Check sheet for the modelled part. Datum: model origin and axes. Units: mm. A direction names the side the tool comes from. Round coordinates to 2 decimals unless told otherwise and drop trailing zeros. Write each loop counter-clockwise with the first axis right and the second up, starting at its lowest first coordinate (ties: lowest second). Pieces come first, ordered by that corner, then holes. Notation, with made-up numbers: M 75,26 L 84,26 A18 ccw 84,54 Z; hole C 28,17.25 d9. An arc over 180 degrees is marked long. Put each result on its own line as item: value.
```python
from build123d import *

# Parameters (mm, degrees)
SKETCH1_W            = 4.8
SKETCH1_H            = 4.8
BOSS_EXTRUDE1_DEPTH  = 20
SKETCH2_W            = 5.2
SKETCH2_H            = 5.2
BOSS_EXTRUDE2_DEPTH  = 50
SKETCH3_W            = 17
SKETCH3_H            = 27
BOSS_EXTRUDE3_DEPTH  = 10
SKETCH4_W            = 13
SKETCH4_H            = 23
CUT_EXTRUDE1_DEPTH   = 8.5
SKETCH5_W            = 11
SKETCH5_H            = 8.5
CUT_EXTRUDE2_DEPTH   = 8.5
SKETCH6_W            = 5
SKETCH6_H            = 5
BOSS_EXTRUDE4_DEPTH  = 81.5
SKETCH7_W            = 5
SKETCH7_H            = 5
BOSS_EXTRUDE5_DEPTH  = 43.1
SKETCH9_R            = 0.9
CUT_EXTRUDE4_DEPTH   = 125.748466924
BOSS_EXTRUDE6_DEPTH  = 5.2
SKETCH13_W           = 17
SKETCH13_H           = 27
BOSS_EXTRUDE7_DEPTH  = 1.5
SKETCH14_W           = 17
SKETCH14_H           = 27
SKETCH14_W_2         = 13
SKETCH14_H_2         = 23
BOSS_EXTRUDE8_DEPTH  = 8.5
SKETCH15_W           = 11
SKETCH15_H           = 8.5
CUT_EXTRUDE6_DEPTH   = 8.5
BOSS_EXTRUDE9_REACH  = 100.782
SKETCH16_W           = 5
SKETCH16_H           = 5
BOSS_EXTRUDE10_DEPTH = 5.2


with BuildPart() as part:
    # Sketch1 → Boss-Extrude1 (new body)
    with BuildSketch(Plane.XY):
        with Locations((2.4, -2.4)):
            Rectangle(SKETCH1_W, SKETCH1_H)
    extrude(amount=BOSS_EXTRUDE1_DEPTH)

    # Sketch2 → Boss-Extrude2 (add)
    with BuildSketch(Plane(origin=(0, 0, 0), x_dir=(-1, 0, 0), z_dir=(0, 0, -1))):
        with Locations((-2.4, -2.4)):
            Rectangle(SKETCH2_W, SKETCH2_H)
    extrude(amount=BOSS_EXTRUDE2_DEPTH)

    # Sketch3 → Boss-Extrude3 (add)
    with BuildSketch(Plane(origin=(0, 0, -50), x_dir=(-1, 0, 0), z_dir=(0, 0, -1))):
        with Locations((-2.4, -2.4)):
            Rectangle(SKETCH3_W, SKETCH3_H)
    extrude(amount=BOSS_EXTRUDE3_DEPTH)

    # Sketch4 → Cut-Extrude1 (cut)
    with BuildSketch(Plane(origin=(0, 0, -60), x_dir=(-1, 0, 0), z_dir=(0, 0, -1))):
        with Locations((-2.4, -2.4)):
            Rectangle(SKETCH4_W, SKETCH4_H)
    extrude(amount=-CUT_EXTRUDE1_DEPTH, mode=Mode.SUBTRACT)

    # Sketch5 → Cut-Extrude2 (cut)
    with BuildSketch(Plane.XZ.offset(15.9)):
        with Locations((2.4, -54.25)):
            Rectangle(SKETCH5_W, SKETCH5_H)
    extrude(amount=-CUT_EXTRUDE2_DEPTH, mode=Mode.SUBTRACT)

    # Sketch6 → Boss-Extrude4 (add)
    with BuildSketch(Plane(origin=(0, 0.2, 0), x_dir=(1, 0, 0), z_dir=(0, 1, 0))):
        with Locations((2.4, 37.5)):
            Rectangle(SKETCH6_W, SKETCH6_H)
    extrude(amount=-BOSS_EXTRUDE4_DEPTH)

    # Sketch7 → Boss-Extrude5 (add)
    with BuildSketch(Plane(origin=(0, 0, -40), x_dir=(-1, 0, 0), z_dir=(0, 0, -1))):
        with Locations((-2.4, -78.8)):
            Rectangle(SKETCH7_W, SKETCH7_H)
    extrude(amount=BOSS_EXTRUDE5_DEPTH)

    # Sketch9 → Cut-Extrude4 (cut, through all)
    with BuildSketch(Plane.XZ.offset(81.3)):
        with Locations((2.4, -80.1)):
            Circle(SKETCH9_R)
    extrude(amount=-CUT_EXTRUDE4_DEPTH, mode=Mode.SUBTRACT)

    # Sketch12 → Boss-Extrude6 (add)
    with BuildSketch(Plane(origin=(5, 0, 0), x_dir=(0, 0, -1), z_dir=(1, 0, 0))):
        Polygon((13.455782968, -5), (35, -40.359932103), (35, -45.359932103), (8.455782968, -5), align=None)
    extrude(amount=-BOSS_EXTRUDE6_DEPTH)


with BuildPart() as body_2:
    # Sketch13 → Boss-Extrude7 (new body)
    with BuildSketch(Plane(origin=(0, -54.71, 0), x_dir=(-1, 0, 0), z_dir=(0, -1, 0))):
        with Locations((-2.6, 15.4)):
            Rectangle(SKETCH13_W, SKETCH13_H)
    extrude(amount=BOSS_EXTRUDE7_DEPTH)

    # Sketch14 → Boss-Extrude8 (add)
    with BuildSketch(Plane.XZ.offset(56.21)):
        with Locations((2.6, -15.4)):
            Rectangle(SKETCH14_W, SKETCH14_H)
        with Locations((2.6, -15.4)):
            Rectangle(SKETCH14_W_2, SKETCH14_H_2, mode=Mode.SUBTRACT)
    extrude(amount=BOSS_EXTRUDE8_DEPTH)

    # Sketch15 → Cut-Extrude6 (cut)
    with BuildSketch(Plane.XY.offset(-1.9)):
        with Locations((2.6, -58.96)):
            Rectangle(SKETCH15_W, SKETCH15_H)
    extrude(amount=-CUT_EXTRUDE6_DEPTH, mode=Mode.SUBTRACT)

    # Sketch16 → Boss-Extrude9 (add, up to next)
    with BuildSketch(Plane.XY.offset(-35), mode=Mode.PRIVATE) as boss_extrude9_sk1:
        with Locations((2.4, -59.859932103)):
            Rectangle(SKETCH16_W, SKETCH16_H)
    boss_extrude9_tool1 = extrude(boss_extrude9_sk1.sketch, amount=BOSS_EXTRUDE9_REACH, mode=Mode.PRIVATE) - body_2.part

    add(part.part)  # Boss-Extrude9 merges part
    add(boss_extrude9_tool1.solids().sort_by_distance((2.4, -59.859932, -35))[0])

    # Sketch18 → Boss-Extrude10 (add)
    with BuildSketch(Plane(origin=(0, 0, 0), x_dir=(0, 0, -1), z_dir=(1, 0, 0))):
        Polygon((25.666047821, -54.71), (5.38231876, -5), (0.38231876, -5), (20.666047821, -54.71), align=None)
    extrude(amount=BOSS_EXTRUDE10_DEPTH)


solid = body_2.part
```
1. Cross-section at D-D (z = 3.5). Enter the section's corners in (x, y), then the cut area to 3 significant figures.
Computed values:
outline: M 0,-4.8 L 4.8,-4.8 L 4.8,0 L 0,0 Z
area: 23.0 mm2
2. Cross-section at B-B (y = -18). Enter the section's corners in (x, z), then the cut area to 3 significant figures.
Computed values:
outline: M -0.2,-21.38 L 5,-21.38 L 5,-17.01 L -0.2,-17.01 Z; M -0.1,-40 L 4.9,-40 L 4.9,-35 L -0.1,-35 Z; M 0,-10.69 L 5.2,-10.69 L 5.2,-5.69 L 0,-5.69 Z
area: 73.7 mm2
3. Depth check by flat-ended pin: pin 1 Ø2.5 at (x, z) = (3.5, 7) entering from -Y; pin 2 Ø1.5 at (x, z) = (1.5, -61) entering from +Y; pin 3 Ø4 at (x, y) = (3.5, -50.5) entering from +Z; pin 4 Ø2 at (x, y) = (-3, -21.5) entering from +Z. Enter the tip coordinate at first touch or a pass-through.
Computed values:
pin 1: stops at y = -4.8
pin 2: stops at y = -76.3
pin 3: stops at z = -18.13
pin 4: passes through
4. Release check for a two-part mould opening along X. For faces 6 (the flat face through (10.9, -3, -55)), 7 (the flat face through (2, -72, -35)), 8 (the flat face through (8.9, -3, -56)), 9 (the flat face through (-5.9, -60, -16)) record: +X half, -X half, draft (parallel to the pull), parting line (faces both ways), or undercut.
Computed values:
face 6: +X half
face 7: draft
face 8: undercut
face 9: -X half
5. Scan lines: probe 1 along Z at (x, y) = (2.4, -77.85); probe 2 along X at (y, z) = (-78.65, -80.1); probe 3 along Z at (x, y) = (3, -13.5). Record each from-to range of solid material in increasing order.
Computed values:
probe 1: z = -83.1 to -81, -79.2 to -35
probe 2: x = -0.1 to 1.5, 3.3 to 4.9
probe 3: z = -40 to -35, -18.63 to -14.05, -8.85 to -3.85
6. Cross-section at C-C (y = -34.5). Enter the section's corners in (x, z).
Computed values:
outline: M -0.2,-31.43 L 5,-31.43 L 5,-27.86 L -0.2,-27.86 Z; M -0.1,-40 L 4.9,-40 L 4.9,-35 L -0.1,-35 Z; M 0,-17.42 L 5.2,-17.42 L 5.2,-12.42 L 0,-12.42 Z
7. Access from +Z, -Z, +X, -X, +Y, -Y to the whole of each face (thin tool, end or side, straight path). Record for faces 1 (the flat face through (2.564, -29.507, -10.382)), 2 (the flat face through (9.1, -60, -16)), 3 (the flat face through (4.8, -2, 10)), 4 (the flat face through (2, -62.36, -32)), 5 (the flat face through (2, -13.9, -59)).
Computed values:
face 1: +Z, +X, -X
face 2: -Y
face 3: +Z, +X, +Y, -Y
face 4: +X, -X, -Y
face 5: -Z
8. Cross-section at A-A (z = -54). Enter the section's corners in (x, y).
Computed values:
outline: M -6.1,-15.9 L -3.1,-15.9 L -3.1,-13.9 L -4.1,-13.9 L -4.1,9.1 L 8.9,9.1 L 8.9,-13.9 L 7.9,-13.9 L 7.9,-15.9 L 10.9,-15.9 L 10.9,11.1 L -6.1,11.1 Z; M -0.1,-81.3 L 4.9,-81.3 L 4.9,-76.3 L -0.1,-76.3 Z
